```python
from build123d import *

# Parameters (mm, degrees)
F1_DEPTH = 25.4
F3_DEPTH = 25.4
F5_DEPTH = 25.4
F7_DEPTH = 25.4
F8_R     = 6.35
F9_DEPTH = 25.4


with BuildPart() as f1:
    # F0 (on Front) → F1 (new body)
    with BuildSketch(Plane.XZ):
        Polygon((0, 38.1), (0, 0), (57.15, 0), (57.15, 12.7), (12.7, 12.7), (12.7, 38.1), align=None)
    extrude(amount=F1_DEPTH)

    # F2 (on face) → F3 (cut)
    with BuildSketch(Plane.YZ.offset(12.7)):
        with BuildLine():
            Line((-25.4, 38.1), (-25.4, 31.75))
            ThreePointArc((-25.4, 31.75), (-12.7, 37.999339), (0, 31.75))
            Line((0, 31.75), (0, 38.1))
            Line((0, 38.1), (-25.4, 38.1))
        make_face()
    extrude(amount=-F3_DEPTH, mode=Mode.SUBTRACT)

    # F4 (on face) → F5 (cut)
    with BuildSketch(Plane.YZ.offset(12.7)):
        with BuildLine():
            ThreePointArc((-6.35, 36.687912), (-12.7, 37.999339), (-19.05, 36.687912))
            Line((-19.05, 36.687912), (-19.05, 30.337912))
            ThreePointArc((-19.05, 30.337912), (-12.7, 23.987912), (-6.35, 30.337912))
            Line((-6.35, 30.337912), (-6.35, 36.687912))
        make_face()
    extrude(amount=-F5_DEPTH, mode=Mode.SUBTRACT)

    # F6 (on face) → F7 (cut)
    with BuildSketch(Plane.XY.offset(12.7)):
        with BuildLine():
            Line((57.15, 0), (50.8, 0))
            ThreePointArc((50.8, 0), (57.099, -12.7), (50.8, -25.4))
            Line((50.8, -25.4), (57.15, -25.4))
            Line((57.15, -25.4), (57.15, 0))
        make_face()
    extrude(amount=-F7_DEPTH, mode=Mode.SUBTRACT)

    # F8 (on face) → F9 (cut)
    with BuildSketch(Plane.XY.offset(12.7)):
        with Locations((25.4, -12.7)):
            Circle(F8_R)
        with Locations((44.399, -12.7)):
            Circle(F8_R)
    extrude(amount=-F9_DEPTH, mode=Mode.SUBTRACT)


solid = f1.part
```
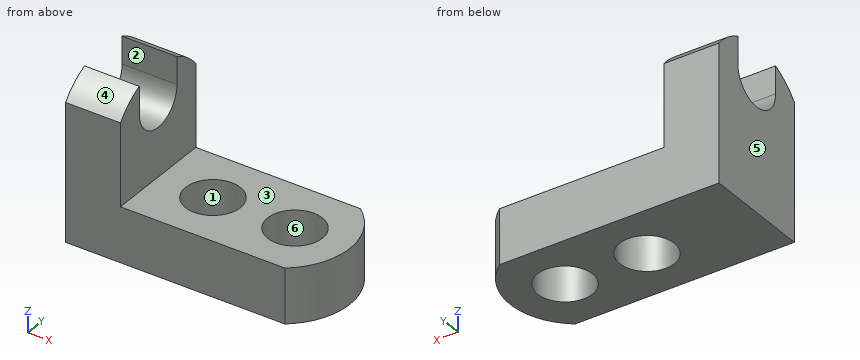
Can you work these out from the model? Positions are in its coordinate system, mm. Face numbers are marked on the shaded views. A direction names the side the tool comes from. Round coordinates to 2 decimals unless told otherwise and drop trailing zeros. Loops run counter-clockwise (first coordinate to the right, second up) from the corner with the lowest first, then second, coordinate; pieces in that order, holes last. Notation, with made-up numbers: (82, -18.75) -> (111, -18.75) arc R19 ccw to (111, 6.25) -> close; hole circle Ø3 at (49, -20). An arc over 180 degrees is marked (long way). Answer in a Markdown table with one row per item.
Item 1: On a 3-axis mill with a long thin cutter (end or side, diameter ignored), from which of +Z, -Z, +X, -X, +Y, -Y can I reach the whole of each face in a straight line? I mean the marked faces 1, 2 and 3. Say none if no direction works.
Answer block:
| item | result |
|---|---|
| face 1 | +Z, -Z |
| face 2 | +Z, +X, -X |
| face 3 | +Z, +X, +Y, -Y |
Item 2: Suppose I cut it at D-D, the plane z = 26. List the corners of the cut face in (x, y) for me.
Answer block:
| item | result |
|---|---|
| outline | (0, -25.4) -> (12.7, -25.4) -> (12.7, -17.34) -> (0, -17.34) -> close; (0, -8.06) -> (12.7, -8.06) -> (12.7, 0) -> (0, 0) -> close |
Item 3: If I drill on probe 1 along Y at (x, z) = (25.4, 6.5); probe 2 along Z at (x, y) = (53, -14.25), over which ranges is the centre line in solid material (lowest first)?
Answer block:
| item | result |
|---|---|
| probe 1 | -25.4 to -19.05, -6.35 to 0 |
| probe 2 | 0 to 12.7 |
Item 4: Will these pins go through, and if not, where does the flat tip stop? P1, Ø12, axis at y = -7, z = 19.5, coming from the +X side; P2, Ø5, axis at y = -12.5, z = 12.5, coming from the +X side; P3, Ø11.5, axis at x = 44.399, y = -12.7, coming from the -Z side.
Answer block:
| item | result |
|---|---|
| P1 | x = 12.7 |
| P2 | x = 57.1 |
| P3 | through |
Item 5: Suppose I cut it at B-B, the plane y = -12.7. List the corners of the cut face in (x, z) for me, plus the area to 3 significant figures.
Answer block:
| item | result |
|---|---|
| outline | (0, 0) -> (19.05, 0) -> (19.05, 12.7) -> (12.7, 12.7) -> (12.7, 23.99) -> (0, 23.99) -> close; (31.75, 0) -> (38.05, 0) -> (38.05, 12.7) -> (31.75, 12.7) -> close; (50.75, 0) -> (57.1, 0) -> (57.1, 12.7) -> (50.75, 12.7) -> close |
| area | 546 mm² |
Item 6: We'd pull the mould along Y, two halves only. Please class the marked faces 4, 5 and 6: released by +Y, released by -Y, zero draft, split by the parting line, or undercut.
Answer block:
| item | result |
|---|---|
| face 4 | released by -Y |
| face 5 | zero draft |
| face 6 | undercut |
Item 7: Suppose I cut it at A-A, the plane x = 25.4. List the corners of the cut face in (y, z) for me, plus the area to 3 significant figures.
Answer block:
| item | result |
|---|---|
| outline | (-25.4, 0) -> (-19.05, 0) -> (-19.05, 12.7) -> (-25.4, 12.7) -> close; (-6.35, 0) -> (0, 0) -> (0, 12.7) -> (-6.35, 12.7) -> close |
| area | 161 mm² |
Item 8: Suppose I cut it at C-C, the plane x = 5. List the corners of the cut face in (y, z) for me, plus the area to 3 significant figures.
Answer block:
| item | result |
|---|---|
| outline | (-25.4, 0) -> (0, 0) -> (0, 31.75) arc R16.03 ccw to (-6.35, 36.69) -> (-6.35, 30.34) arc R6.35 cw to (-19.05, 30.34) -> (-19.05, 36.69) arc R16.03 ccw to (-25.4, 31.75) -> close |
| area | 762 mm² |
